Geometry: see drawing. Coordinates: mm, zero at the bounding-box minimum. Round coordinates to 2 decimals unless told otherwise and drop trailing zeros. Write each loop counter-clockwise with the first axis right and the second up, starting at its lowest first coordinate (ties: lowest second). Pieces come first, ordered by that corner, then holes. Notation, with made-up numbers: M 25,12 L 50,12 A25 ccw 50,24 Z; hole C 22,-31.75 d10. An arc over 180 degrees is marked long. Use a Markdown table: item, result.
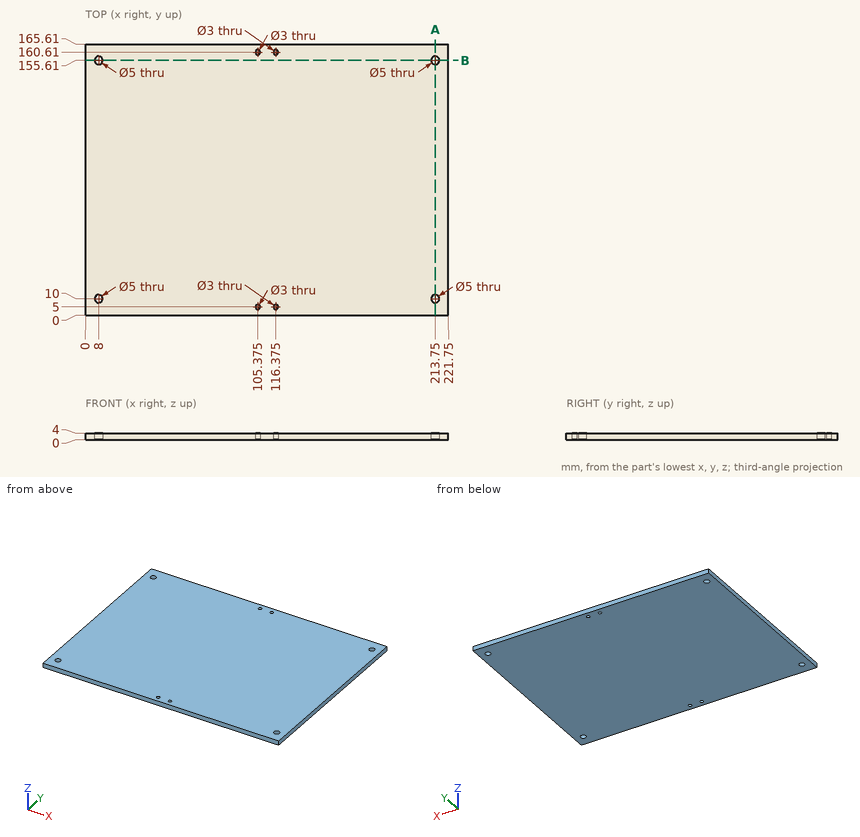
Q1. Section A-A on x = 213.75. Return loops of the section in (y, z), plus the area to 3 significant figures.
Results are:
| item | result |
|---|---|
| outline | M 0,0 L 7.5,0 L 7.5,4 L 0,4 Z; M 12.5,0 L 153.11,0 L 153.11,4 L 12.5,4 Z; M 158.11,0 L 165.61,0 L 165.61,4 L 158.11,4 Z |
| area | 622 mm^2 |
Q2. Section B-B on y = 155.61. Return loops of the section in (x, z), plus the area to 3 significant figures.
Results are:
| item | result |
|---|---|
| outline | M 0,0 L 5.5,0 L 5.5,4 L 0,4 Z; M 10.5,0 L 211.25,0 L 211.25,4 L 10.5,4 Z; M 216.25,0 L 221.75,0 L 221.75,4 L 216.25,4 Z |
| area | 847 mm^2 |
Q3. Line query: L1, parallel to Y at x = 8, z = 1.15. Output: solid intervals per line, ascending.
Results are:
| item | result |
|---|---|
| L1 | 0 to 7.5, 12.5 to 153.11, 158.11 to 165.61 |
Q4. First-contact query: pin 1 Ø1.8 at (x, y) = (105.375, 5) entering from -Z. Flat tip, straight axial feed; report the tip coordinate or a pass-through.
Results are:
| item | result |
|---|---|
| pin 1 | through |
